from build123d import *

# Parameters (mm, degrees)
SKETCH1_R           = 31.75
BOSS_EXTRUDE3_DEPTH = 10.16
SKETCH3_R           = 27.94
CUT_EXTRUDE1_DEPTH  = 2.54
SKETCH4_R           = 3.175
CUT_EXTRUDE2_DEPTH  = 46.543269536
CUT_EXTRUDE3_DEPTH  = 46.543269536
CUT_EXTRUDE4_DEPTH  = 46.543269536
FILLET1_R           = 2.54


with BuildPart() as part:
    # Sketch1 → Boss-Extrude3 (new body)
    with BuildSketch(Plane(origin=(0, 0, 0), x_dir=(1, 0, 0), z_dir=(0, 1, 0))):
        with Locations(Location((0, 0, 0), (0, 0, 270))):
            Circle(SKETCH1_R)
    extrude(amount=BOSS_EXTRUDE3_DEPTH)

    # Sketch3 → Cut-Extrude1 (cut)
    with BuildSketch(Plane(origin=(0, 10.16, 0), x_dir=(1, 0, 0), z_dir=(0, 1, 0))):
        with Locations(Location((0, 0, 0), (0, 0, 270))):
            Circle(SKETCH3_R)
    extrude(amount=-CUT_EXTRUDE1_DEPTH, mode=Mode.SUBTRACT)

    # Sketch4 → Cut-Extrude2 (cut, through all)
    with BuildSketch(Plane(origin=(0, 7.62, 0), x_dir=(1, 0, 0), z_dir=(0, 1, 0))):
        with Locations(Location((0, 0, 0), (0, 0, 270))):
            Circle(SKETCH4_R)
    extrude(amount=-CUT_EXTRUDE2_DEPTH, mode=Mode.SUBTRACT)

    # Sketch5 → Cut-Extrude3 (cut, through all)
    with BuildSketch(Plane(origin=(0, 7.62, 0), x_dir=(1, 0, 0), z_dir=(0, 1, 0))):
        with BuildLine():
            Line((12.39620867, 9.285356697), (18.617912617, 10.952457245))
            ThreePointArc((18.617912617, 10.952457245), (20.413963841, 12.748508469), (19.756563466, 15.201960068))
            Line((19.756563466, 15.201960068), (15.201960068, 19.756563466))
            ThreePointArc((15.201960068, 19.756563466), (12.748508469, 20.413963841), (10.952457245, 18.617912617))
            Line((10.952457245, 18.617912617), (9.285356697, 12.39620867))
            ThreePointArc((9.285356697, 12.39620867), (9.942757071, 9.942757071), (12.39620867, 9.285356697))
        make_face()
        with BuildLine():
            Line((9.285356697, -12.39620867), (10.952457245, -18.617912617))
            ThreePointArc((10.952457245, -18.617912617), (12.748508469, -20.413963841), (15.201960068, -19.756563466))
            Line((15.201960068, -19.756563466), (19.756563466, -15.201960068))
            ThreePointArc((19.756563466, -15.201960068), (20.413963841, -12.748508469), (18.617912617, -10.952457245))
            Line((18.617912617, -10.952457245), (12.39620867, -9.285356697))
            ThreePointArc((12.39620867, -9.285356697), (9.942757071, -9.942757071), (9.285356697, -12.39620867))
        make_face()
        with BuildLine():
            Line((-12.39620867, -9.285356697), (-18.617912617, -10.952457245))
            ThreePointArc((-18.617912617, -10.952457245), (-20.413963841, -12.748508469), (-19.756563466, -15.201960068))
            Line((-19.756563466, -15.201960068), (-15.201960068, -19.756563466))
            ThreePointArc((-15.201960068, -19.756563466), (-12.748508469, -20.413963841), (-10.952457245, -18.617912617))
            Line((-10.952457245, -18.617912617), (-9.285356697, -12.39620867))
            ThreePointArc((-9.285356697, -12.39620867), (-9.942757071, -9.942757071), (-12.39620867, -9.285356697))
        make_face()
        with BuildLine():
            Line((-9.285356697, 12.39620867), (-10.952457245, 18.617912617))
            ThreePointArc((-10.952457245, 18.617912617), (-12.748508469, 20.413963841), (-15.201960068, 19.756563466))
            Line((-15.201960068, 19.756563466), (-19.756563466, 15.201960068))
            ThreePointArc((-19.756563466, 15.201960068), (-20.413963841, 12.748508469), (-18.617912617, 10.952457245))
            Line((-18.617912617, 10.952457245), (-12.39620867, 9.285356697))
            ThreePointArc((-12.39620867, 9.285356697), (-9.942757071, 9.942757071), (-9.285356697, 12.39620867))
        make_face()
        with BuildLine():
            Line((-3.81, 19.05), (-3.81, 34.374285303))
            Line((-3.81, 34.374285303), (3.81, 34.374285303))
            Line((3.81, 34.374285303), (3.81, 19.05))
            ThreePointArc((3.81, 19.05), (0, 15.24), (-3.81, 19.05))
        make_face()
    extrude(amount=-CUT_EXTRUDE3_DEPTH, mode=Mode.SUBTRACT)

    # Sketch5<2> → Cut-Extrude4 (cut, through all)
    with BuildSketch(Plane(origin=(0, 7.62, 0), x_dir=(1, 0, 0), z_dir=(0, 1, 0))):
        with BuildLine():
            Line((12.39620867, 9.285356697), (18.617912617, 10.952457245))
            ThreePointArc((18.617912617, 10.952457245), (20.413963841, 12.748508469), (19.756563466, 15.201960068))
            Line((19.756563466, 15.201960068), (15.201960068, 19.756563466))
            ThreePointArc((15.201960068, 19.756563466), (12.748508469, 20.413963841), (10.952457245, 18.617912617))
            Line((10.952457245, 18.617912617), (9.285356697, 12.39620867))
            ThreePointArc((9.285356697, 12.39620867), (9.942757071, 9.942757071), (12.39620867, 9.285356697))
        make_face()
        with BuildLine():
            Line((9.285356697, -12.39620867), (10.952457245, -18.617912617))
            ThreePointArc((10.952457245, -18.617912617), (12.748508469, -20.413963841), (15.201960068, -19.756563466))
            Line((15.201960068, -19.756563466), (19.756563466, -15.201960068))
            ThreePointArc((19.756563466, -15.201960068), (20.413963841, -12.748508469), (18.617912617, -10.952457245))
            Line((18.617912617, -10.952457245), (12.39620867, -9.285356697))
            ThreePointArc((12.39620867, -9.285356697), (9.942757071, -9.942757071), (9.285356697, -12.39620867))
        make_face()
        with BuildLine():
            Line((-12.39620867, -9.285356697), (-18.617912617, -10.952457245))
            ThreePointArc((-18.617912617, -10.952457245), (-20.413963841, -12.748508469), (-19.756563466, -15.201960068))
            Line((-19.756563466, -15.201960068), (-15.201960068, -19.756563466))
            ThreePointArc((-15.201960068, -19.756563466), (-12.748508469, -20.413963841), (-10.952457245, -18.617912617))
            Line((-10.952457245, -18.617912617), (-9.285356697, -12.39620867))
            ThreePointArc((-9.285356697, -12.39620867), (-9.942757071, -9.942757071), (-12.39620867, -9.285356697))
        make_face()
        with BuildLine():
            Line((-9.285356697, 12.39620867), (-10.952457245, 18.617912617))
            ThreePointArc((-10.952457245, 18.617912617), (-12.748508469, 20.413963841), (-15.201960068, 19.756563466))
            Line((-15.201960068, 19.756563466), (-19.756563466, 15.201960068))
            ThreePointArc((-19.756563466, 15.201960068), (-20.413963841, 12.748508469), (-18.617912617, 10.952457245))
            Line((-18.617912617, 10.952457245), (-12.39620867, 9.285356697))
            ThreePointArc((-12.39620867, 9.285356697), (-9.942757071, 9.942757071), (-9.285356697, 12.39620867))
        make_face()
        with BuildLine():
            Line((-3.81, 19.05), (-3.81, 34.374285303))
            Line((-3.81, 34.374285303), (3.81, 34.374285303))
            Line((3.81, 34.374285303), (3.81, 19.05))
            ThreePointArc((3.81, 19.05), (0, 15.24), (-3.81, 19.05))
        make_face()
    extrude(amount=CUT_EXTRUDE4_DEPTH, mode=Mode.SUBTRACT)

    # Loft4: read off the stored shape, not the designer's step
    # Loft4: loft between two sections, ruled curve by curve
    loft4_from = [
        Edge.make_bspline([(21.644950372, 15.24, 2.885330399), (15.874289575, 15.24, 5.535231144), (13.22438883, 15.24, -0.235429654), (18.995049628, 15.24, -2.885330399), (24.765710425, 15.24, -5.535231144), (27.41561117, 15.24, 0.235429654), (21.644950372, 15.24, 2.885330399)], [0, 0, 0, 0, 0.5, 0.5, 0.5, 1, 1, 1, 1], 3, [1, 0.333333333, 0.333333333, 1, 0.333333333, 0.333333333, 1]),
    ]
    loft4_to = [
        Edge.make_bspline([(21.092187722, 7.62, 3.079667372), (14.932852978, 7.62, 4.624042816), (13.388477534, 7.62, -1.535291928), (19.547812278, 7.62, -3.079667372), (25.707147022, 7.62, -4.624042816), (27.251522466, 7.62, 1.535291928), (21.092187722, 7.62, 3.079667372)], [0, 0, 0, 0, 0.5, 0.5, 0.5, 1, 1, 1, 1], 3, [1, 0.333333333, 0.333333333, 1, 0.333333333, 0.333333333, 1]),
    ]
    loft4 = Solid(Shell([*[Face.make_surface_from_curves(loft4_from[k], loft4_to[k]) for k in range(1)], Face(Wire(loft4_from)), Face(Wire(loft4_to))]))
    add(loft4)

    # Fillet1
    fillet1_edges = [part.edges().sort_by_distance(p)[0] for p in [
        (19.547812278, 7.62, -3.079667372),
    ]]
    fillet(fillet1_edges, radius=FILLET1_R)


solid = part.part
Read the model definition and answer for the solid it produces. Units are mm, in the model's axes. A direction names the side the tool comes from. Coordinates: 2 decimals unless noted, no trailing zeros. Loops run counter-clockwise (first coordinate to the right, second up) from the corner with the lowest first, then second, coordinate; pieces in that order, holes last.
Q1. The part is cut by section B-B on y = 2.25. Give the number of separate pieces and of enclosed holes in the cut face, and give its area (3 significant figures).
Q2. The mould has two halves that part along X. Classify faces 4 (the face through (12.785, 3.863, -20.423)), 5 (the face through (21, 10.16, 19)): +X half, -X half, draft (parallel to the pull), parting line (faces both ways), or undercut.
Q3. Which of the six approach directions +Z, -Z, +X, -X, +Y, -Y give full straight-line access (tool end or side, diameter ignored) to faces 1 (the face through (20, 15.24, 0)), 2 (the face through (-10.107, 3.863, -15.464)), 3 (the face through (-3.81, 4, -25))?
Q4. Each of these flat-tipped pins is pushed along its axis until it touches: pin 1 Ø2 at (x, y) = (18, 2) entering from -Z; pin 2 Ø4 at (y, z) = (9, -20) entering from -X; pin 3 Ø1 at (x, y) = (1.5, 6.5) entering from -Z; pin 4 Ø1 at (y, z) = (11.5, -4.5) entering from +X. Where does it stop, or does it pass through?
Q5. The part is cut by section C-C on x = 1.5. Write down the section's boundary in (y, z), and give its area (3 significant figures).
Q6. The part is cut by section A-A on z = -14. Write down the section's boundary in (x, y), and give its area (3 significant figures).
Q7. The part is cut by section D-D on z = 23. Write down the section's boundary in (x, y).
Q8. Consider probe 1 along X at (y, z) = (4.75, 0) (3 decimals); probe 2 along X at (y, z) = (8.45, 0); probe 3 along X at (y, z) = (8.6, 0). Determine where each line is inside the solid, lowest interval first.
Results below:
1. separate pieces: 1
1. enclosed holes: 5
1. area: 2,670 mm2
2. face 4: undercut
2. face 5: draft
3. face 1: +Z, -Z, +X, -X, +Y
3. face 2: +Y, -Y
3. face 3: -Z, +Y, -Y
4. pin 1: stops at z = -26.82
4. pin 2: stops at x = -26.15
4. pin 3: stops at z = -15.81
4. pin 4: passes through
5. outline: (0, -15.55) - (7.62, -15.55) - (7.62, -2.8) - (0, -2.8) - close; (0, 2.8) - (7.62, 2.8) - (7.62, 27.9) - (10.16, 27.9) - (10.16, 31.71) - (0, 31.71) - close
5. area: 327 mm2
6. outline: (-28.5, 0) - (-20.43, 0) - (-20.43, 7.62) - (-24.18, 7.62) - (-24.18, 10.16) - (-28.5, 10.16) - close; (-9.72, 0) - (9.72, 0) - (9.72, 7.62) - (-9.72, 7.62) - close; (20.43, 0) - (28.5, 0) - (28.5, 10.16) - (24.18, 10.16) - (24.18, 7.62) - (20.43, 7.62) - close
6. area: 293 mm2
7. outline: (-21.89, 0) - (21.89, 0) - (21.89, 10.16) - (15.86, 10.16) - (15.86, 7.62) - (-15.86, 7.62) - (-15.86, 10.16) - (-21.89, 10.16) - close
8. probe 1: x = -31.75 to -3.175, 3.175 to 31.75
8. probe 2: x = -31.75 to -27.94, 16.5 to 24.14, 27.94 to 31.75
8. probe 3: x = -31.75 to -27.94, 16.62 to 24.02, 27.94 to 31.75
